Verification items for the finished model (mm, model axes). A direction names the side the tool comes from. Give positions to 0.01 mm unless a question says otherwise; leave off trailing zeros. Loops run counter-clockwise (first coordinate to the right, second up) from the corner with the lowest first, then second, coordinate; pieces in that order, holes last. Notation, with made-up numbers: M 58,82 L 65,82 A3 ccw 65,86 Z; hole C 23.5,86.5 d7. An arc over 180 degrees is marked long. Use a Markdown table: item, result.
from build123d import *

# Parameters (mm, degrees)
BOSS_EXTRUDE1_DEPTH     = 110
CUT_EXTRUDE1_DEPTH      = 114.495594628
CUT_EXTRUDE1_DEPTH_BACK = 30
SKETCH5_R               = 25
SKETCH5_R_2             = 12.5
BOSS_EXTRUDE2_DEPTH     = 100
CUT_EXTRUDE2_DEPTH      = 170.852877515
CUT_EXTRUDE2_DEPTH_BACK = 170.852877515
SKETCH6_W               = 32.203850694
SKETCH6_H               = 7
CUT_EXTRUDE3_DEPTH      = 170.670177936
CUT_EXTRUDE3_DEPTH_BACK = 170.670177936
SKETCH7_R               = 12.5


with BuildPart() as part:
    # Sketch1 → Boss-Extrude1 (new body)
    with BuildSketch(Plane.YZ):
        with BuildLine():
            ThreePointArc((10, 12.5), (0, 2.5), (-10, 12.5))
            Line((-10, 12.5), (-25, 12.5))
            Line((-25, 12.5), (-25, -12.5))
            Line((-25, -12.5), (25, -12.5))
            Line((25, -12.5), (25, 12.5))
            Line((25, 12.5), (10, 12.5))
        make_face()
        with BuildLine():
            Line((10, 12.5), (-10, 12.5))
            ThreePointArc((-10, 12.5), (0, 2.5), (10, 12.5))
        make_face()
    extrude(amount=-BOSS_EXTRUDE1_DEPTH)

    # Sketch4 → Cut-Extrude1 (cut, two sides: drawn at the far end of the back side and taken through both)
    with BuildSketch(Plane.YZ.offset(-CUT_EXTRUDE1_DEPTH_BACK)):
        with BuildLine():
            Line((-10, 12.5), (10, 12.5))
            ThreePointArc((10, 12.5), (0, 2.5), (-10, 12.5))
        make_face()
    extrude(amount=CUT_EXTRUDE1_DEPTH + CUT_EXTRUDE1_DEPTH_BACK, mode=Mode.SUBTRACT)

    # Sketch5 → Boss-Extrude2 (add)
    with BuildSketch(Plane(origin=(0, 0, -12.5), x_dir=(1, 0, 0), z_dir=(0, 0, -1))):
        with Locations(Location((-110, 0, 0), (0, 0, 270))):
            Circle(SKETCH5_R)
        with Locations(Location((-110, 0, 0), (0, 0, 270))):
            Circle(SKETCH5_R_2, mode=Mode.SUBTRACT)
    extrude(amount=-BOSS_EXTRUDE2_DEPTH)

    # Sketch6 → Cut-Extrude2 (cut, two sides: drawn at the far end of the back side and taken through both)
    with BuildSketch(Plane.XY.offset(87.5).offset(-CUT_EXTRUDE2_DEPTH_BACK)):
        with Locations((-126.101925347, -0.117088635)):
            Rectangle(SKETCH6_W, SKETCH6_H)
    extrude(amount=CUT_EXTRUDE2_DEPTH + CUT_EXTRUDE2_DEPTH_BACK, mode=Mode.SUBTRACT)

    # Sketch7 → Cut-Extrude3 (cut, two sides: drawn at the far end of the back side and taken through both)
    with BuildSketch(Plane.XY.offset(87.5).offset(-CUT_EXTRUDE3_DEPTH_BACK)):
        with Locations((-110, 0)):
            Circle(SKETCH7_R)
    extrude(amount=CUT_EXTRUDE3_DEPTH + CUT_EXTRUDE3_DEPTH_BACK, mode=Mode.SUBTRACT)


solid = part.part
(1) Cross-section at A-A on y = -7.5. Record the cut outline in (x, z), then the cut area to 3 significant figures.
Results below:
| item | result |
|---|---|
| outline | M -133.85,-12.5 L -120,-12.5 L -120,87.5 L -133.85,87.5 Z; M -100,-12.5 L 0,-12.5 L 0,5.89 L -30,5.89 L -30,12.5 L -86.15,12.5 L -86.15,87.5 L -100,87.5 Z |
| area | 4,730 mm^2 |
(2) Material ranges on line 1 (Y direction, x = -110, z = 67.5); line 2 (Z direction, x = -74.5, y = 10.5); line 3 (X direction, y = 9, z = 23.5), recorded low to high.
Results below:
| item | result |
|---|---|
| line 1 | -25 to -12.5, 12.5 to 25 |
| line 2 | -12.5 to 12.5 |
| line 3 | -133.32 to -118.67, -101.33 to -86.68 |
(3) Set-up check for faces 1 (the flat face through (-98, -6, 87.5)), 2 (the flat face through (-54, 25, 0)), 3 (the flat face through (-128, -3.617, 37)), 4 (the cylindrical face through (-132.753, 10.358, 36.8)), 5 (the cylindrical face through (-15.2, 0.2, 2.5)): record each of +Z, -Z, +X, -X, +Y, -Y from which the full face is reachable in a straight line by a thin tool's end or side.
Results below:
| item | result |
|---|---|
| face 1 | +Z, +X, -X, +Y, -Y |
| face 2 | +Z, -Z, +X, -X, +Y |
| face 3 | +Z, -Z, -X |
| face 4 | +Z |
| face 5 | +Z, +X |
(4) Gauge pin test, flat ends, axial feed: P1, Ø15, axis at x = -110, y = 0, coming from the -Z side; P2, Ø4, axis at x = -128.5, z = 43.5, coming from the -Y side; P3, Ø8, axis at y = -3.5, z = 10, coming from the +X side; P4, Ø12, axis at x = -67, y = -8, coming from the +Z side. Record the tip position at first contact, or that the pin passes through.
Results below:
| item | result |
|---|---|
| P1 | through |
| P2 | y = -18.78 |
| P3 | x = -30 |
| P4 | z = 12.5 |
(5) Cross-section at C-C on x = -27. Record the cut outline in (y, z), then the cut area to 3 significant figures.
Results below:
| item | result |
|---|---|
| outline | M -25,-12.5 L 25,-12.5 L 25,12.5 L 10,12.5 A10 cw -10,12.5 L -25,12.5 Z |
| area | 1,090 mm^2 |
(6) Cross-section at D-D on y = 0. Record the cut outline in (x, z).
Results below:
| item | result |
|---|---|
| outline | M -97.5,-12.5 L 0,-12.5 L 0,2.5 L -30,2.5 L -30,12.5 L -85,12.5 L -85,87.5 L -97.5,87.5 Z |
(7) Cross-section at B-B on z = -5.5. Record the cut outline in (x, y), then the cut area to 3 significant figures.
Results below:
| item | result |
|---|---|
| outline | M -134.77,3.38 L -122.03,3.38 A12.5 cw long -121.97,-3.62 L -134.74,-3.62 A25 ccw -110,-25 L 0,-25 L 0,25 L -110,25 A25 ccw Z |
| area | 5,900 mm^2 |
(8) Draft check along X on faces 6 (the cylindrical face through (-97.515, 0.622, 36.8)), 7 (the flat face through (0, 0, 0)), 8 (the flat face through (-128, 3.383, 37)). Enter one of: +X half, -X half, draft (parallel to the pull), parting line (faces both ways), or undercut.
Results below:
| item | result |
|---|---|
| face 6 | undercut |
| face 7 | +X half |
| face 8 | draft |
